Geometry check sheet. Reference: the model listing, model coordinates, mm. A direction names the side the tool comes from. Coordinates: 2 decimals unless noted, no trailing zeros. Write each loop counter-clockwise with the first axis right and the second up, starting at its lowest first coordinate (ties: lowest second). Pieces come first, ordered by that corner, then holes. Notation, with made-up numbers: M 61,28 L 115,28 A19 cw 115,62 Z; hole C 86.5,-17.75 d4. An arc over 180 degrees is marked long. Put each result on its own line as item: value. Start each with the question number.
1) Scan lines: line 1 along X through (y, z) = (7.4, -6.5); line 2 along Z through (x, y) = (-1, 9.35); line 3 along X through (y, z) = (8.15, -2). Record each from-to range of solid material in increasing order.
2) Set-up check for faces 5 (the flat face through (1.2, 9.92, -5.3)), 6 (the flat face through (0, 6, -7.95)), 7 (the flat face through (1.004, 8, -5)), 8 (the flat face through (-2.846, 9, -5)), 9 (the flat face through (4, 8.093, -5)): record each of +Z, -Z, +X, -X, +Y, -Y from which the full face is reachable in a straight line by a thin tool's end or side.
3) Cross-section at A-A on z = -6. Record the cut outline in (x, y), plus the area to 3 significant figures.
4) Mould release check, pull along X, two halves, no side actions. Record for faces 1 (the flat face through (5.277, 7, -5)), 2 (the flat face through (0, 7, -10.2)), 3 (the flat face through (-4.446, 5.729, -5.27)), 4 (the flat face through (0, 8, -3.45)): released by +X, released by -X, zero draft, split by the parting line, or undercut.
5) Gauge pin test, flat ends, axial feed: pin 1 (1 mm diameter, centred on y = 5.5, z = -6, fed in from -X); pin 2 (1.2 mm diameter, centred on x = -0.5, z = -6.5, fed in from -Y); pin 3 (2.5 mm diameter, centred on x = -4, z = -3, fed in from +Y); pin 4 (0.9 mm diameter, centred on y = 9, z = -4, fed in from -X). Record the tip position at first contact, or that the pin passes through.
6) Cross-section at B-B on x = -0.5. Record the cut outline in (y, z), plus the area to 3 significant figures.
7) Cross-section at D-D on z = -8.25. Record the cut outline in (x, y).
8) Cross-section at C-C on y = 7.5. Record the cut outline in (x, z), plus the area to 3 significant figures.
from build123d import *

# Parameters (mm, degrees)
PAD_DEPTH       = 10
SKETCH002_W     = 2.5
SKETCH002_H     = 5.5
POCKET_DEPTH    = 2
SKETCH003_W     = 2.254226
SKETCH003_H     = 3.5
POCKET001_DEPTH = 5


with BuildPart() as part:
    # Sketch001 → Pad (new body)
    with BuildSketch(Plane.XY):
        Polygon((5.277013, 8.093206), (5.277013, 6.560121), (3.637013, 4.920121), (-3.637013, 4.920121), (-5.277013, 6.560121), (-5.277013, 8.093206), (-2.845653, 8.093206), (-2.845653, 9.920121), (2.845653, 9.920121), (2.845653, 8.093206), align=None)
    extrude(amount=PAD_DEPTH)

    # Sketch002 (on Face3 of Pad) → Pocket (cut)
    with BuildSketch(Plane.XZ.offset(-4.920121)):
        with Locations((0, 5)):
            Rectangle(SKETCH002_W, SKETCH002_H)
    extrude(amount=-POCKET_DEPTH, mode=Mode.SUBTRACT)

    # Sketch003 (on Face17 of Pocket) → Pocket001 (cut)
    with BuildSketch(Plane.XZ.offset(-6.920121)):
        with Locations((-0.122887, 5)):
            Rectangle(SKETCH003_W, SKETCH003_H)
    extrude(amount=-POCKET001_DEPTH, mode=Mode.SUBTRACT)


with BuildPart() as part_1:
    # Body placement: moved
    add(part.part.moved(Location((0, 0, -10.2))))


solid = part_1.part
Answer key:
1. line 1: x = -5.28 to -1.25, 1 to 5.28
1. line 2: z = -10.2 to -6.95, -3.45 to -0.2
1. line 3: x = -2.85 to 2.85
2. face 5: +Z, -Z, +X, -X, +Y
2. face 6: -Y
2. face 7: +Y, -Y
2. face 8: +Z, -Z, -X, +Y
2. face 9: +Z, -Z, +X, +Y
3. outline: M -5.28,6.56 L -3.64,4.92 L -1.25,4.92 L -1.25,9.92 L -2.85,9.92 L -2.85,8.09 L -5.28,8.09 Z; M 1,6.92 L 1.25,6.92 L 1.25,4.92 L 3.64,4.92 L 5.28,6.56 L 5.28,8.09 L 2.85,8.09 L 2.85,9.92 L 1,9.92 Z
3. area: 29.4 mm²
4. face 1: released by +X
4. face 2: zero draft
4. face 3: released by -X
4. face 4: undercut
5. pin 1: stops at x = -4.72
5. pin 2: stops at y = 6.92
5. pin 3: stops at y = 9.92
5. pin 4: stops at x = -2.85
6. outline: M 4.92,-10.2 L 9.92,-10.2 L 9.92,-6.95 L 6.92,-6.95 L 6.92,-7.95 L 4.92,-7.95 Z; M 4.92,-2.45 L 6.92,-2.45 L 6.92,-3.45 L 9.92,-3.45 L 9.92,-0.2 L 4.92,-0.2 Z
6. area: 28.5 mm²
7. outline: M -5.28,6.56 L -3.64,4.92 L 3.64,4.92 L 5.28,6.56 L 5.28,8.09 L 2.85,8.09 L 2.85,9.92 L -2.85,9.92 L -2.85,8.09 L -5.28,8.09 Z
8. outline: M -5.28,-10.2 L 5.28,-10.2 L 5.28,-0.2 L -5.28,-0.2 Z; hole M -1.25,-6.95 L 1,-6.95 L 1,-3.45 L -1.25,-3.45 Z
8. area: 97.7 mm²
